from build123d import *

# Parameters (mm, degrees)
SKETCH2_W           = 175
SKETCH2_H           = 100
BOSS_EXTRUDE1_DEPTH = 75
SKETCH3_W           = 40
SKETCH3_H           = 22
CUT_EXTRUDE1_DEPTH  = 30
SKETCH4_W           = 40
SKETCH4_H           = 22
BOSS_EXTRUDE2_DEPTH = 25


with BuildPart() as part:
    # Sketch2 → Boss-Extrude1 (new body)
    with BuildSketch(Plane(origin=(0, 0, 0), x_dir=(1, 0, 0), z_dir=(0, 1, 0))):
        Rectangle(SKETCH2_W, SKETCH2_H)
    extrude(amount=BOSS_EXTRUDE1_DEPTH)

    # Sketch3 → Cut-Extrude1 (cut)
    with BuildSketch(Plane.XZ):
        with Locations((-67.5, 39)):
            Rectangle(SKETCH3_W, SKETCH3_H)
        with Locations((67.5, 39)):
            Rectangle(SKETCH3_W, SKETCH3_H)
        with Locations((-67.5, -39)):
            Rectangle(SKETCH3_W, SKETCH3_H)
        with Locations((67.5, -39)):
            Rectangle(SKETCH3_W, SKETCH3_H)
    extrude(amount=-CUT_EXTRUDE1_DEPTH, mode=Mode.SUBTRACT)

    # Sketch4 → Boss-Extrude2 (add)
    with BuildSketch(Plane(origin=(0, 75, 0), x_dir=(1, 0, 0), z_dir=(0, 1, 0))):
        with Locations((-67.5, 39)):
            Rectangle(SKETCH4_W, SKETCH4_H)
        with Locations((67.5, 39)):
            Rectangle(SKETCH4_W, SKETCH4_H)
        with Locations((67.5, -39)):
            Rectangle(SKETCH4_W, SKETCH4_H)
        with Locations((-67.5, -39)):
            Rectangle(SKETCH4_W, SKETCH4_H)
    extrude(amount=BOSS_EXTRUDE2_DEPTH)


solid = part.part
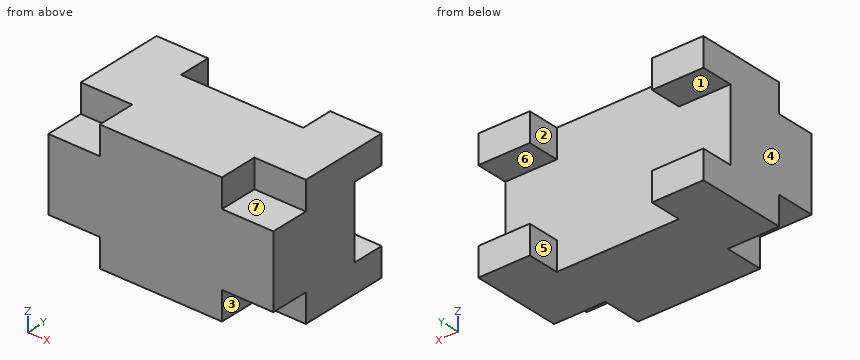
CAD build for the part. Positions are in the model's coordinates, mm. Face numbers are marked on the shaded views. A direction names the side the tool comes from. Give positions to 0.01 mm unless a question says otherwise; leave off trailing zeros. Order: outer loops, then holes, each group sorted by start corner. A loop starts at its lowest first (then second) coordinate and runs counter-clockwise, first axis right, second up. Notation, with made-up numbers: (57.25, 15) - (71.25, 15) arc R34 ccw to (71.25, 54) - close; hole circle Ø7 at (-13, 51). An arc over 180 degrees is marked (long way). Answer in a Markdown table with one row per item.
1. Saw through at D-D, the plane x = 44.5. Give the cut face in (y, z), plus the area to 3 significant figures.
Data:
| item | result |
|---|---|
| outline | (0, -50) - (75, -50) - (75, 50) - (0, 50) - close |
| area | 7,500 mm² |
2. Saw through at B-B, the plane z = -40.5. Give the cut face in (x, y).
Data:
| item | result |
|---|---|
| outline | (-87.5, 30) - (-47.5, 30) - (-47.5, 0) - (47.5, 0) - (47.5, 30) - (87.5, 30) - (87.5, 100) - (47.5, 100) - (47.5, 75) - (-47.5, 75) - (-47.5, 100) - (-87.5, 100) - close |
3. Saw through at C-C, the plane y = 12.5. Give the cut face in (x, z).
Data:
| item | result |
|---|---|
| outline | (-87.5, -28) - (-47.5, -28) - (-47.5, -50) - (47.5, -50) - (47.5, -28) - (87.5, -28) - (87.5, 28) - (47.5, 28) - (47.5, 50) - (-47.5, 50) - (-47.5, 28) - (-87.5, 28) - close |
4. Saw through at A-A, the plane y = 91. Give the cut face in (x, z), plus the area to 3 significant figures.
Data:
| item | result |
|---|---|
| outline | (-87.5, -50) - (-47.5, -50) - (-47.5, -28) - (-87.5, -28) - close; (-87.5, 28) - (-47.5, 28) - (-47.5, 50) - (-87.5, 50) - close; (47.5, -50) - (87.5, -50) - (87.5, -28) - (47.5, -28) - close; (47.5, 28) - (87.5, 28) - (87.5, 50) - (47.5, 50) - close |
| area | 3,520 mm² |
5. Flat gauge pins, fed straight in: pin 1 (15 mm diameter, centred on x = -74, y = 22, fed in from +Z); pin 2 (11 mm diameter, centred on y = 15.5, z = 35, fed in from +X); pin 3 (5 mm diameter, centred on x = -1.5, z = 25, fed in from +Y). Where does each tip first touch, or does it go through?
Data:
| item | result |
|---|---|
| pin 1 | stops at z = 28 |
| pin 2 | stops at x = 47.5 |
| pin 3 | stops at y = 75 |
6. Pull direction X, two halves, no side cores. Call the marked faces 1, 2, 3 and 4: pulls with the +X half, pulls with the -X half, needs draft (parallel to the pull), parting line crosses it, or undercut.
Data:
| item | result |
|---|---|
| face 1 | needs draft |
| face 2 | undercut |
| face 3 | pulls with the +X half |
| face 4 | pulls with the -X half |
7. Probe probe 1 along Y at (x, z) = (60.5, -27.5); probe 2 along Z at (x, y) = (67, 25.5); probe 3 along Y at (x, z) = (59, 28.5). List the from-to ranges inside material, lowest first. Write a range as [from, to].
Data:
| item | result |
|---|---|
| probe 1 | y = [0, 75] |
| probe 2 | z = [-28, 28] |
| probe 3 | y = [30, 100] |
8. Tool access for the marked faces 5, 6 and 7: list every direction of +Z, -Z, +X, -X, +Y, -Y with a clear straight run to the whole face (end or side of a thin tool).
Data:
| item | result |
|---|---|
| face 5 | +Z, -Z, +Y |
| face 6 | +X, -X, +Y |
| face 7 | +Z, +X, -Y |
